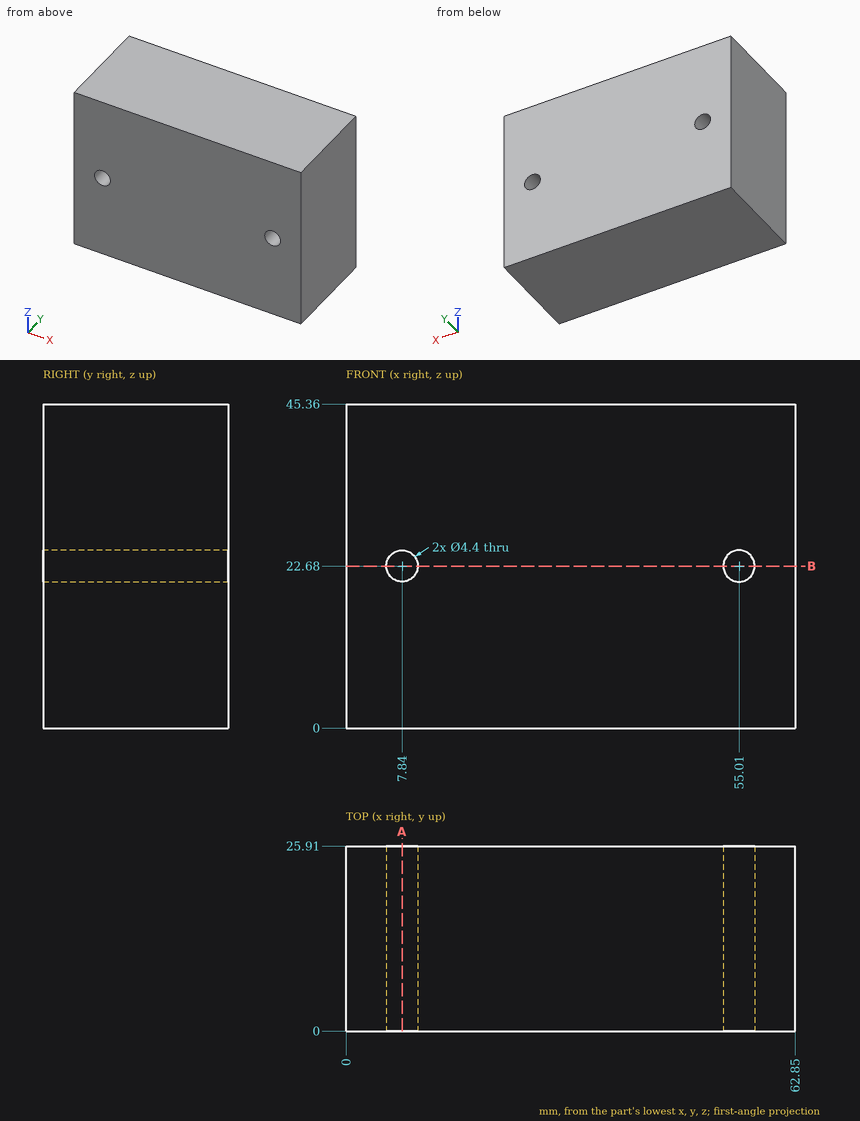
Input: dimensioned drawing with shaded views. Units: mm. Origin: part minimum x, y, z. Give positions to 0.01 mm unless a question says otherwise; leave off trailing zeros. Order: outer loops, then holes, each group sorted by start corner. A loop starts at its lowest first (then second) coordinate and runs counter-clockwise, first axis right, second up. Notation, with made-up numbers: (84.5, -40) -> (113.5, -40) arc R20 cw to (113.5, -6) -> close; hole circle Ø10 at (45.25, 11.25). An arc over 180 degrees is marked (long way). Use a Markdown table: item, result.
1) Contact query for a flat-ended pin moving along its axis: P1, Ø1, axis at x = 23, y = 6, coming from the -Z side. Output: stop coordinate, or through.
Answer list:
| item | result |
|---|---|
| P1 | z = 0 |
2) Section query A-A, the plane x = 7.84. Return the cut outline in (y, z).
Answer list:
| item | result |
|---|---|
| outline | (0, 0) -> (25.91, 0) -> (25.91, 20.48) -> (0, 20.48) -> close; (0, 24.88) -> (25.91, 24.88) -> (25.91, 45.36) -> (0, 45.36) -> close |
3) Ray query, line 1 along X through (y, z) = (12, 22.68); line 2 along Z through (x, y) = (7.84, 16.5). Return the intervals inside material, ascending. Write a range as [from, to].
Answer list:
| item | result |
|---|---|
| line 1 | [0, 5.64], [10.04, 52.81], [57.21, 62.85] |
| line 2 | [0, 20.48], [24.88, 45.36] |
4) Section query B-B, the plane z = 22.68. Return the cut outline in (x, y).
Answer list:
| item | result |
|---|---|
| outline | (0, 0) -> (5.64, 0) -> (5.64, 25.91) -> (0, 25.91) -> close; (10.04, 0) -> (52.81, 0) -> (52.81, 25.91) -> (10.04, 25.91) -> close; (57.21, 0) -> (62.85, 0) -> (62.85, 25.91) -> (57.21, 25.91) -> close |
